Read the model definition and answer for the solid it produces. Units are mm, in the model's axes. A direction names the side the tool comes from. Coordinates: 2 decimals unless noted, no trailing zeros. Loops run counter-clockwise (first coordinate to the right, second up) from the corner with the lowest first, then second, coordinate; pieces in that order, holes last.
from build123d import *

# Parameters (mm, degrees)
SKETCH1_W                    = 100
SKETCH1_H                    = 50
BASE_FLANGE1_DEPTH           = 3
SKETCH2_R                    = 11.05
SKETCH2_R_2                  = 1.75
CUT_EXTRUDE1_DEPTH           = 104.121287812
SKETCH3_R                    = 1.75
CUT_EXTRUDE2_DEPTH           = 104.121287812
CIRPATTERN1_COUNT            = 4
CUT_EXTRUDE3_DEPTH           = 104.121287812
SKETCHED_BEND2_OUTLINE_W     = 3
SKETCHED_BEND2_OUTLINE_H     = 50
SKETCHED_BEND2_DEPTH         = 47.020021532
SKETCHED_START               = 47.383443248
SKETCHED_BEND2_2_OUTLINE_W   = 47.979978468
SKETCHED_BEND2_2_OUTLINE_H   = 50
SKETCHED_BEND2_2_OUTLINE_R   = 1.75
SKETCHED_BEND2_2_OUTLINE_R_2 = 11.05
SKETCHED_BEND2_2_DEPTH       = 2.636578284
SKETCHED_START_2             = 47.020021532
SKETCHED_BEND2_3_OUTLINE_W   = 47.979978468
SKETCHED_BEND2_3_OUTLINE_H   = 50
SKETCHED_BEND2_3_OUTLINE_R   = 1.75
SKETCHED_BEND2_3_OUTLINE_R_2 = 11.05
SKETCHED_BEND2_3_DEPTH       = 3.7366
SKETCHED_START_3             = -26
SKETCHED_BEND2_4_DEPTH       = 52
BOSS_EXTRUDE1_DEPTH          = 3
CHAMFER1_SIZE                = 5
CHAMFER2_SIZE                = 0.3
CHAMFER3_SIZE                = 0.3
SKETCH7_R                    = 3
CUT_EXTRUDE4_DEPTH           = 1.5


with BuildPart() as part:
    # Base-Flange1: sheet metal written as solids
    # Sketch1 → Base-Flange1 (new body)
    with BuildSketch(Plane(origin=(0, 0, 0), x_dir=(1, 0, 0), z_dir=(0, 1, 0))):
        with Locations((50, 0)):
            Rectangle(SKETCH1_W, SKETCH1_H)
    extrude(amount=-BASE_FLANGE1_DEPTH)

    # Sketch2 → Cut-Extrude1 (cut, through all)
    with BuildSketch(Plane(origin=(0, 0, 0), x_dir=(1, 0, 0), z_dir=(0, 1, 0))):
        with Locations(Location((21, 0, 0), (0, 0, 270))):
            Circle(SKETCH2_R)
        with Locations(Location((5.5, 15.5, 0), (0, 0, 270))):
            Circle(SKETCH2_R_2)
        with Locations(Location((36.5, 15.5, 0), (0, 0, 270))):
            Circle(SKETCH2_R_2)
        with Locations(Location((36.5, -15.5, 0), (0, 0, 270))):
            Circle(SKETCH2_R_2)
        with Locations(Location((5.5, -15.5, 0), (0, 0, 270))):
            Circle(SKETCH2_R_2)
    extrude(amount=-CUT_EXTRUDE1_DEPTH, mode=Mode.SUBTRACT)

    # Sketch3 → Cut-Extrude2 (cut, through all)
    with BuildSketch(Plane(origin=(0, 0, 0), x_dir=(1, 0, 0), z_dir=(0, 1, 0))):
        with Locations(Location((11.100505063, 9.899494937, 0), (0, 0, 270))):
            Circle(SKETCH3_R)
    cut_extrude2 = extrude(amount=-CUT_EXTRUDE2_DEPTH, mode=Mode.SUBTRACT)

    # CirPattern1: Cut-Extrude2 ×4 about axis
    cirpattern1_axis = Axis((21, 0, 0), (0, 1, 0))
    for i in range(1, CIRPATTERN1_COUNT):
        add(cut_extrude2.rotate(cirpattern1_axis, i * 360 / CIRPATTERN1_COUNT), mode=Mode.SUBTRACT)

    # Sketch4 → Cut-Extrude3 (cut, through all)
    with BuildSketch(Plane(origin=(0, 0, 0), x_dir=(1, 0, 0), z_dir=(0, 1, 0))):
        with BuildLine():
            Line((59, 17.1), (89, 17.1))
            ThreePointArc((89, 17.1), (91.1, 15), (89, 12.9))
            Line((89, 12.9), (59, 12.9))
            ThreePointArc((59, 12.9), (56.9, 15), (59, 17.1))
        make_face()
        with BuildLine():
            Line((59, -12.9), (89, -12.9))
            ThreePointArc((89, -12.9), (91.1, -15), (89, -17.1))
            Line((89, -17.1), (59, -17.1))
            ThreePointArc((59, -17.1), (56.9, -15), (59, -12.9))
        make_face()
    extrude(amount=-CUT_EXTRUDE3_DEPTH, mode=Mode.SUBTRACT)

    # Sketched Bend2: read off the stored shape, not the designer's step
    # Sketched Bend2 outline → Sketched Bend2 (cut)
    with BuildSketch(Plane.YZ):
        with Locations((-1.5, 0)):
            Rectangle(SKETCHED_BEND2_OUTLINE_W, SKETCHED_BEND2_OUTLINE_H)
    extrude(amount=SKETCHED_BEND2_DEPTH, mode=Mode.SUBTRACT)

    # Sketched Bend2 2 outline → Sketched Bend2 2 (add)
    with BuildSketch(Plane.YZ.offset(SKETCHED_START)):
        with Locations((23.989989234, 0)):
            Rectangle(SKETCHED_BEND2_2_OUTLINE_W, SKETCHED_BEND2_2_OUTLINE_H)
        with Locations((11.479978468, -15.5)):
            Circle(SKETCHED_BEND2_2_OUTLINE_R, mode=Mode.SUBTRACT)
        with Locations((17.080483531, -9.899494937)):
            Circle(SKETCHED_BEND2_2_OUTLINE_R, mode=Mode.SUBTRACT)
        with Locations((42.479978468, -15.5)):
            Circle(SKETCHED_BEND2_2_OUTLINE_R, mode=Mode.SUBTRACT)
        with Locations((36.879473404, -9.899494937)):
            Circle(SKETCHED_BEND2_2_OUTLINE_R, mode=Mode.SUBTRACT)
        with Locations((17.080483531, 9.899494937)):
            Circle(SKETCHED_BEND2_2_OUTLINE_R, mode=Mode.SUBTRACT)
        with Locations((11.479978468, 15.5)):
            Circle(SKETCHED_BEND2_2_OUTLINE_R, mode=Mode.SUBTRACT)
        with Locations((26.979978468, 0)):
            Circle(SKETCHED_BEND2_2_OUTLINE_R_2, mode=Mode.SUBTRACT)
        with Locations((36.879473404, 9.899494937)):
            Circle(SKETCHED_BEND2_2_OUTLINE_R, mode=Mode.SUBTRACT)
        with Locations((42.479978468, 15.5)):
            Circle(SKETCHED_BEND2_2_OUTLINE_R, mode=Mode.SUBTRACT)
    extrude(amount=SKETCHED_BEND2_2_DEPTH)

    # Sketched Bend2 3 outline → Sketched Bend2 3 (add)
    with BuildSketch(Plane.YZ.offset(SKETCHED_START_2)):
        with Locations((23.989989234, 0)):
            Rectangle(SKETCHED_BEND2_3_OUTLINE_W, SKETCHED_BEND2_3_OUTLINE_H)
        with Locations((11.479978468, -15.5)):
            Circle(SKETCHED_BEND2_3_OUTLINE_R, mode=Mode.SUBTRACT)
        with Locations((17.080483531, -9.899494937)):
            Circle(SKETCHED_BEND2_3_OUTLINE_R, mode=Mode.SUBTRACT)
        with Locations((42.479978468, -15.5)):
            Circle(SKETCHED_BEND2_3_OUTLINE_R, mode=Mode.SUBTRACT)
        with Locations((36.879473404, -9.899494937)):
            Circle(SKETCHED_BEND2_3_OUTLINE_R, mode=Mode.SUBTRACT)
        with Locations((17.080483531, 9.899494937)):
            Circle(SKETCHED_BEND2_3_OUTLINE_R, mode=Mode.SUBTRACT)
        with Locations((11.479978468, 15.5)):
            Circle(SKETCHED_BEND2_3_OUTLINE_R, mode=Mode.SUBTRACT)
        with Locations((26.979978468, 0)):
            Circle(SKETCHED_BEND2_3_OUTLINE_R_2, mode=Mode.SUBTRACT)
        with Locations((36.879473404, 9.899494937)):
            Circle(SKETCHED_BEND2_3_OUTLINE_R, mode=Mode.SUBTRACT)
        with Locations((42.479978468, 15.5)):
            Circle(SKETCHED_BEND2_3_OUTLINE_R, mode=Mode.SUBTRACT)
    extrude(amount=SKETCHED_BEND2_3_DEPTH)

    # Sketched Bend2 4 outline → Sketched Bend2 4 (cut)
    with BuildSketch(Plane.XY.offset(SKETCHED_START_3)):
        with BuildLine():
            Line((50.756621532, 47.979978468), (50.020021532, 47.979978468))
            Line((50.020021532, 47.979978468), (50.020021532, 0.7366))
            ThreePointArc((50.020021532, 0.7366), (50.235766677, 0.215745145), (50.756621532, 0))
            Line((50.756621532, 0), (50.756621532, 47.979978468))
        make_face()
        with BuildLine():
            ThreePointArc((50.756621532, -3), (48.114446333, -1.905575198), (47.020021532, 0.7366))
            Line((47.020021532, 0.7366), (47.020021532, -3))
            Line((47.020021532, -3), (50.756621532, -3))
        make_face()
    extrude(amount=SKETCHED_BEND2_4_DEPTH, mode=Mode.SUBTRACT)

    # Sketch6 → Boss-Extrude1 (add)
    with BuildSketch(Plane.XY.offset(25)):
        Polygon((50.020021532, 20), (63.020021532, 0), (52.020021532, 0), (50.020021532, 3.076923077), align=None)
    boss_extrude1 = extrude(amount=-BOSS_EXTRUDE1_DEPTH)

    # Mirror1: Boss-Extrude1 across plane
    add(boss_extrude1.mirror(Plane.XY))

    # Chamfer1
    chamfer1_edges = [part.edges().sort_by_distance(p)[0] for p in [
        (100, -1.5, -25),
        (100, -1.5, 25),
        (48.520021532, 47.979978468, -25),
        (48.520021532, 47.979978468, 25),
    ]]
    chamfer(chamfer1_edges, length=CHAMFER1_SIZE)

    # Chamfer2
    chamfer2_edges = [part.edges().sort_by_distance(p)[0] for p in [
        (74, 0, -17.1),
        (91.1, 0, -15),
        (74, 0, -12.9),
        (56.9, 0, -15),
        (74, 0, 12.9),
        (91.1, 0, 15),
        (74, 0, 17.1),
        (56.9, 0, 15),
        (56.9, -3, 15),
        (74, -3, 17.1),
        (91.1, -3, 15),
        (74, -3, 12.9),
        (56.9, -3, -15),
        (74, -3, -12.9),
        (91.1, -3, -15),
        (74, -3, -17.1),
        (47.020021532, 15.929978468, 0),
        (50.020021532, 15.929978468, 0),
        (47.020021532, 40.729978468, -15.5),
        (50.020021532, 40.729978468, -15.5),
        (47.020021532, 9.729978468, -15.5),
        (50.020021532, 9.729978468, -15.5),
        (47.020021532, 9.729978468, 15.5),
        (50.020021532, 9.729978468, 15.5),
        (47.020021532, 40.729978468, 15.5),
        (50.020021532, 40.729978468, 15.5),
    ]]
    chamfer(chamfer2_edges, length=CHAMFER2_SIZE)

    # Chamfer3
    chamfer3_edges = [part.edges().sort_by_distance(p)[0] for p in [
        (47.020021532, 35.129473404, -9.899494937),
        (50.020021532, 35.129473404, -9.899494937),
        (47.020021532, 35.129473404, 9.899494937),
        (50.020021532, 35.129473404, 9.899494937),
        (47.020021532, 15.330483531, 9.899494937),
        (50.020021532, 15.330483531, 9.899494937),
        (47.020021532, 15.330483531, -9.899494937),
        (50.020021532, 15.330483531, -9.899494937),
    ]]
    chamfer(chamfer3_edges, length=CHAMFER3_SIZE)

    # Sketch7 → Cut-Extrude4 (cut)
    with BuildSketch(Plane(origin=(0, 0, 0), x_dir=(1, 0, 0), z_dir=(0, 1, 0))):
        with Locations((86, -15)):
            Circle(SKETCH7_R)
        with Locations((62, -15)):
            Circle(SKETCH7_R)
        with Locations((86, 15)):
            Circle(SKETCH7_R)
        with Locations((62, 15)):
            Circle(SKETCH7_R)
    extrude(amount=-CUT_EXTRUDE4_DEPTH, mode=Mode.SUBTRACT)


solid = part.part
Q1. A cutting plane is placed at A-A (z = 0). Give the vertices of the cut face in (x, y).
Findings below:
outline: (47.02, 0.74) arc R3.74 ccw to (50.76, -3) - (100, -3) - (100, 0) - (50.76, 0) arc R0.74 cw to (50.02, 0.74) - (50.02, 15.63) - (49.72, 15.93) - (47.32, 15.93) - (47.02, 15.63) - close; (47.02, 38.33) - (47.32, 38.03) - (49.72, 38.03) - (50.02, 38.33) - (50.02, 47.98) - (47.02, 47.98) - close
Q2. Straight lines are drawn through the part: probe 1 along Y at (x, z) = (48.25, 15.5); probe 2 along Y at (x, z) = (49, 15.5); probe 3 along Y at (x, z) = (85, -1). For each, find the intervals that lie inside material, in ascending order.
Findings below:
probe 1: y = -2.03 to 9.73, 13.23 to 40.73, 44.23 to 47.98
probe 2: y = -2.56 to 9.73, 13.23 to 40.73, 44.23 to 47.98
probe 3: y = -3 to 0
Q3. A cutting plane is placed at B-B (x = 68). Give the vertices of the cut face in (y, z), then the cut area to 3 significant figures.
Findings below:
outline: (-3, -25) - (0, -25) - (0, -17.4) - (-0.3, -17.1) - (-2.7, -17.1) - (-3, -17.4) - close; (-3, -12.6) - (-2.7, -12.9) - (-0.3, -12.9) - (0, -12.6) - (0, 12.6) - (-0.3, 12.9) - (-2.7, 12.9) - (-3, 12.6) - close; (-3, 17.4) - (-2.7, 17.1) - (-0.3, 17.1) - (0, 17.4) - (0, 25) - (-3, 25) - close
area: 124 mm2
Q4. Flat-ended cylindrical pins translate along their axes: pin 1 Ø0.7 at (x, z) = (87, 17.5) entering from +Y; pin 2 Ø0.5 at (x, z) = (85, -17.5) entering from +Y; pin 3 Ø5.5 at (y, z) = (17.08, -9.9) entering from +X. Find the tip coordinate at first contact, or state that the pin passes through.
Findings below:
pin 1: stops at y = 0
pin 2: stops at y = -1.5
pin 3: stops at x = 50.02
Q5. Determine the mould class of faces 3 (the face through (56.43, 10.14, -23.52)), 4 (the face through (48.503, 43.421, 16.976)), 5 (the face through (62, -1, -12)) for opening direction X: +X half, -X half, draft (parallel to the pull), parting line (faces both ways), or undercut.
Findings below:
face 3: +X half
face 4: draft
face 5: undercut
Q6. A cutting plane is placed at C-C (y = 36). Count the separate pieces of the cut face and the enclosed holes in it, then the cut area to 3 significant figures.
Findings below:
separate pieces: 4
enclosed holes: 0
area: 92.8 mm2
Q7. Which of the six approach directions +Z, -Z, +X, -X, +Y, -Y give full straight-line access (tool end or side, diameter ignored) to faces 1 (the face through (48.503, 12.421, -14.024)), 2 (the face through (62, -1, 12))?
Findings below:
face 1: +X, -X
face 2: +Y
